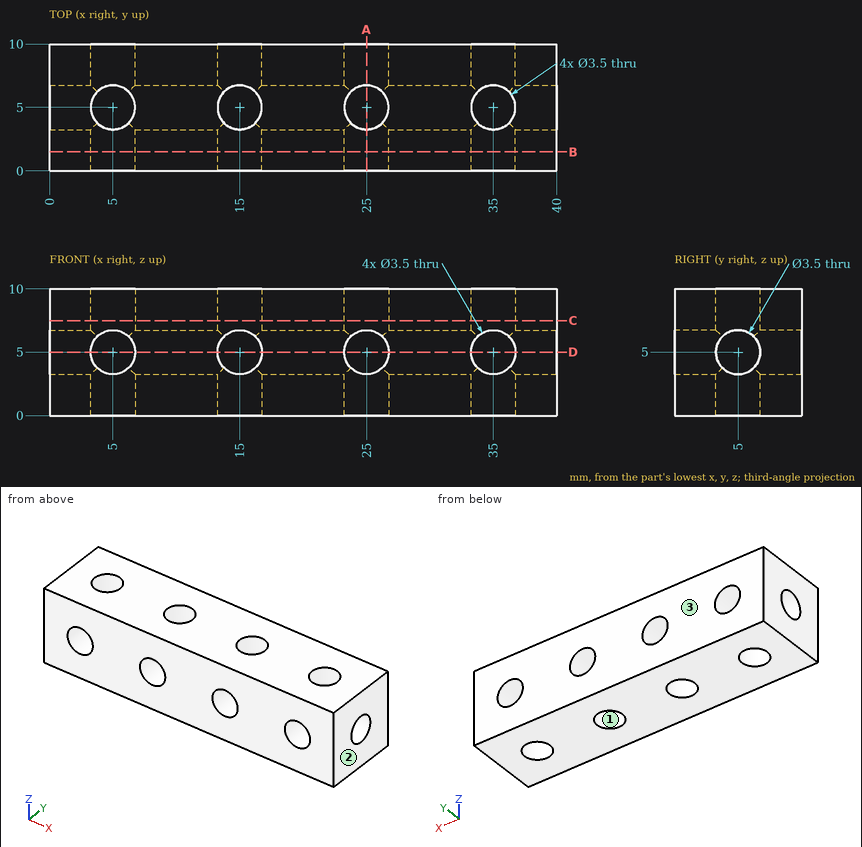
Can you work these out from the drawing? Everything is in mm from the part's minimum corner. Round coordinates to 2 decimals unless told otherwise and drop trailing zeros. Order: outer loops, then holes, each group sorted by start corner. A loop starts at its lowest first (then second) coordinate and runs counter-clockwise, first axis right, second up.
(1) I'm going to push a flat-ended pin straight in: pin 1 (3 mm diameter, centred on y = 5, z = 5, fed in from -X). Where does the tip first touch, or does it pass through?
Results are:
pin 1: passes through
(2) We'd pull the mould along Y, two halves only. Please class the marked faces 1, 2 and 3: +Y half, -Y half, draft (parallel to the pull), parting line (faces both ways), or undercut.
Results are:
face 1: undercut
face 2: draft
face 3: +Y half
(3) If we section it at A-A (x = 25): Please give me the cut outline in (y, z).
Results are:
outline: (0, 0) - (3.25, 0) - (3.25, 3.25) - (0, 3.25) - close; (0, 6.75) - (3.25, 6.75) - (3.25, 10) - (0, 10) - close; (6.75, 0) - (10, 0) - (10, 3.25) - (6.75, 3.25) - close; (6.75, 6.75) - (10, 6.75) - (10, 10) - (6.75, 10) - close
(4) If we section it at B-B (y = 1.5): Please give me the cut outline in (x, z).
Results are:
outline: (0, 0) - (40, 0) - (40, 10) - (0, 10) - close; hole circle Ø3.5 at (5, 5); hole circle Ø3.5 at (15, 5); hole circle Ø3.5 at (25, 5); hole circle Ø3.5 at (35, 5)
(5) If I drill on L1, parallel to X at y = 5, z = 1.9; L2, parallel to Y at x = 15, z = 8.85; L3, parallel to X at y = 8.75, z = 3.5, over which ranges is the centre line in solid material (lowest first)?
Results are:
L1: x = 0 to 3.25, 6.75 to 13.25, 16.75 to 23.25, 26.75 to 33.25, 36.75 to 40
L2: y = 0 to 3.25, 6.75 to 10
L3: x = 0 to 4.1, 5.9 to 14.1, 15.9 to 24.1, 25.9 to 34.1, 35.9 to 40
(6) If we section it at D-D (z = 5): Count the separate pieces of the cut face and the enclosed holes in it, plus the area to 3 significant figures.
Results are:
separate pieces: 10
enclosed holes: 0
area: 169 mm2
